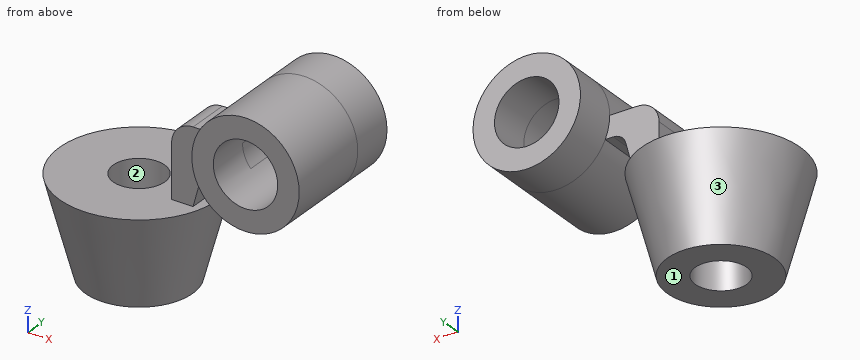
from build123d import *

# Parameters (mm, degrees)
SKETCH3_W                = 10
SKETCH3_H                = 25
SKETCH3_H_2              = 10
BOSS_EXTRUDE1_DEPTH      = 10
FILLET1_R                = 6
FILLET2_R                = 10
SKETCH4_R                = 15
CUT_EXTRUDE1_DEPTH       = 48
SKETCH4_3_R              = 25
SKETCH4_3_R_2            = 15
BOSS_EXTRUDE2_DEPTH      = 20
BOSS_EXTRUDE2_DEPTH_BACK = 40


with BuildPart() as part:
    # Sketch1 → Revolve1 (revolve)
    with BuildSketch(Plane(origin=(0, 0, 0), x_dir=(1, 0, 0), z_dir=(0, 1, 0))):
        Polygon((12, 45), (0, 0), (25, 0), (25, 45), align=None)
    revolve(axis=Axis((37, 0, 0), (0, 0, -1)))

    # Sketch3 → Boss-Extrude1 (add, symmetric)
    with BuildSketch(Plane(origin=(0, 0, 0), x_dir=(1, 0, 0), z_dir=(0, 1, 0))):
        with Locations((64, -12.5)):
            Rectangle(SKETCH3_W, SKETCH3_H)
        with Locations((64, -30)):
            Rectangle(SKETCH3_W, SKETCH3_H_2)
        Polygon((75.698729811, -25), (69, -25), (69, -35), (107, -35), (107, -25), align=None)
        Polygon((75.698729811, -25), (69, 0), (69, -25), align=None)
    extrude(amount=BOSS_EXTRUDE1_DEPTH, both=True)

    # Fillet1
    fillet1_edges = [part.edges().sort_by_distance(p)[0] for p in [
        (75.698729811, 0, 25),
    ]]
    fillet(fillet1_edges, radius=FILLET1_R)

    # Fillet2
    fillet2_edges = [part.edges().sort_by_distance(p)[0] for p in [
        (59, 0, 35),
    ]]
    fillet(fillet2_edges, radius=FILLET2_R)

    # Sketch4 → Cut-Extrude1 (cut, through all)
    with BuildSketch(Plane(origin=(0, 10, 0), x_dir=(1, 0, 0), z_dir=(0, 1, 0))):
        with Locations((107, -35)):
            Circle(SKETCH4_R)
    extrude(amount=-CUT_EXTRUDE1_DEPTH, mode=Mode.SUBTRACT)

    # Sketch4_3 → Boss-Extrude2 (add, two sides)
    with BuildSketch(Plane(origin=(0, 10, 0), x_dir=(1, 0, 0), z_dir=(0, 1, 0))) as boss_extrude2_sk:
        with Locations((107, -35)):
            Circle(SKETCH4_3_R)
        with Locations((107, -35)):
            Circle(SKETCH4_3_R_2, mode=Mode.SUBTRACT)
    extrude(amount=BOSS_EXTRUDE2_DEPTH)
    extrude(boss_extrude2_sk.sketch, amount=-BOSS_EXTRUDE2_DEPTH_BACK)


solid = part.part
Can you work these out from the model? Positions are in its coordinate system, mm. Face numbers are marked on the shaded views. Coordinates: 2 decimals unless noted, no trailing zeros. Write each loop counter-clockwise with the first axis right and the second up, starting at its lowest first coordinate (ties: lowest second). Pieces come first, ordered by that corner, then holes. Notation, with made-up numbers: (-28.75, 51.5) -> (7.25, 51.5) arc R28 cw to (7.25, 69.5) -> close; hole circle Ø3 at (4.5, -20.75). An arc over 180 degrees is marked (long way). Answer as CSV lines item,"result".
1) Will these pins go through, and if not, where does the flat tip stop? P1, Ø10, axis at y = 4, z = 10, coming from the -X side; P2, Ø6.5, axis at x = 78, y = 4, coming from the +Z side; P3, Ø7.5, axis at x = 72.5, z = 25.5, coming from the -Y side.
Check result:
P1,"x = 59"
P2,"z = 35"
P3,"y = -10"
2) If we section it at B-B on x = 37: Please give me the cut outline in (y, z).
Check result:
outline,"(-37, 0) -> (-25, -45) -> (-12, -45) -> (-12, 0) -> close; (12, -45) -> (25, -45) -> (37, 0) -> (12, 0) -> close"
3) If I drill on line 1 (X direction, y = 23, z = 35); line 2 (Z direction, x = 107, y = 24.25); line 3 (Z direction, x = 37, y = 13), over which ranges is the centre line in solid material (lowest first)? Write a range as from..to.
Check result:
line 1,"82..92, 122..132"
line 2,"10..20, 50..60"
line 3,"-45..0"
4) If we section it at A-A on y = 0: Please give me the cut outline in (x, z), then the cut area to 3 significant figures.
Check result:
outline,"(0, 0) -> (12, -45) -> (25, -45) -> (25, 0) -> close; (49, -45) -> (62, -45) -> (74, 0) -> (69, 0) -> (74.51, 20.55) arc R6 cw to (80.3, 25) -> (84.09, 25) arc R25 ccw (long way) to (82, 35) -> (69, 35) arc R10 ccw to (59, 25) -> (59, 0) -> (49, 0) -> close; hole circle Ø30 at (107, 35)"
area,"3,520 mm²"
5) If we section it at C-C on x = 107: Please give me the cut outline in (y, z), then the cut area to 3 significant figures.
Check result:
outline,"(-30, 10) -> (30, 10) -> (30, 20) -> (-30, 20) -> close; (-30, 50) -> (30, 50) -> (30, 60) -> (-30, 60) -> close"
area,"1,200 mm²"
6) If we section it at D-D on z = 6: Please give me the cut outline in (x, y).
Check result:
outline,"(59, -10) -> (70.61, -10) -> (70.61, 10) -> (59, 10) -> close"
7) If we mould it in two halves opening along X, with no side actions, what happens to the marked faces 1, 2 and 3? For each: +X half, -X half, draft (parallel to the pull), parting line (faces both ways), or undercut.
Check result:
face 1,"draft"
face 2,"undercut"
face 3,"parting line"
